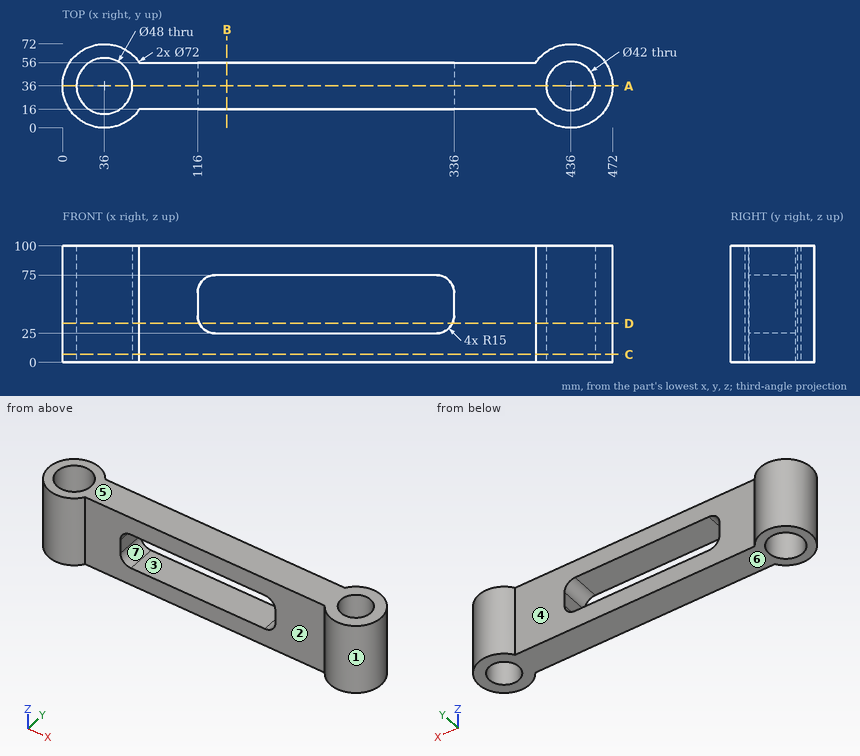
Source: three-view drawing plus pictorial views. Frame: mm from the lowest corner of the part. A direction names the side the tool comes from. Round coordinates to 2 decimals unless told otherwise and drop trailing zeros. Loops run counter-clockwise (first coordinate to the right, second up) from the corner with the lowest first, then second, coordinate; pieces in that order, holes last.
Item 1: Section B-B, the plane x = 141. Output: boundary loops of the cut face in (y, z).
Checked values:
outline: (16, 0) - (56, 0) - (56, 25) - (16, 25) - close; (16, 75) - (56, 75) - (56, 100) - (16, 100) - close
Item 2: Section D-D, the plane z = 33.5. Output: boundary loops of the cut face in (x, y).
Checked values:
outline: (65.93, 16) - (117.48, 16) - (117.48, 56) - (65.93, 56) arc R36 ccw (long way) to start; (334.52, 16) - (406.07, 16) arc R36 ccw (long way) to (406.07, 56) - (334.52, 56) - close; hole circle Ø48 at (36, 36); hole circle Ø42 at (436, 36)
Item 3: Contact query for flat-ended pins moving along their axis: P1, Ø8, axis at x = 422.5, z = 31, coming from the +Y side; P2, Ø16, axis at y = 27.5, z = 50.5, coming from the +X side; P3, Ø5, axis at y = 22, z = 34.5, coming from the +X side. Output: stop coordinate, or through.
Checked values:
P1: stops at y = 70.72
P2: stops at x = 472
P3: stops at x = 470.11
Item 4: Mould query, pull axis Z, two halves, no side actions, for the marked faces 4, 5, 6 and 7. Classes: released by +Z, released by -Z, zero draft, split by the parting line, or undercut.
Checked values:
face 4: zero draft
face 5: released by +Z
face 6: released by -Z
face 7: undercut
Item 5: Section C-C, the plane z = 7. Output: boundary loops of the cut face in (x, y), plus the area to 3 significant figures.
Checked values:
outline: (65.93, 16) - (406.07, 16) arc R36 ccw (long way) to (406.07, 56) - (65.93, 56) arc R36 ccw (long way) to start; hole circle Ø48 at (36, 36); hole circle Ø42 at (436, 36)
area: 18,200 mm2
Item 6: Section A-A, the plane y = 36. Output: boundary loops of the cut face in (x, z), plus the area to 3 significant figures.
Checked values:
outline: (0, 0) - (12, 0) - (12, 100) - (0, 100) - close; (60, 0) - (415, 0) - (415, 100) - (60, 100) - close; (457, 0) - (472, 0) - (472, 100) - (457, 100) - close; hole (116, 40) arc R15 ccw to (131, 25) - (321, 25) arc R15 ccw to (336, 40) - (336, 60) arc R15 ccw to (321, 75) - (131, 75) arc R15 ccw to (116, 60) - close
area: 27,400 mm2
Item 7: Line query: L1, parallel to X at y = 36, z = 56; L2, parallel to X at y = 36, z = 79; L3, parallel to Y at x = 36, z = 31. Output: solid intervals per line, ascending.
Checked values:
L1: x = 0 to 12, 60 to 116, 336 to 415, 457 to 472
L2: x = 0 to 12, 60 to 415, 457 to 472
L3: y = 0 to 12, 60 to 72
Item 8: Reachability of the marked faces 1, 2 and 3 from +Z, -Z, +X, -X, +Y, -Y: full face, straight path, thin tool, end or side. Return the list, or none.
Checked values:
face 1: +Z, -Z
face 2: +Z, -Z, -Y
face 3: +Y, -Y
